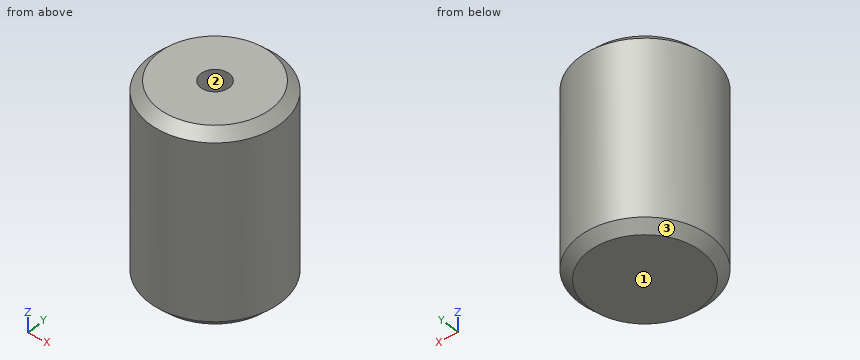
from build123d import *

# Parameters (mm, degrees)
F0_R     = 13.5
F1_DEPTH = 40
F2_R     = 2.9
F3_DEPTH = 35
F4_SIZE  = 2


with BuildPart() as f1:
    # F0 (on Top) → F1 (new body)
    with BuildSketch(Plane.XY):
        Circle(F0_R)
    extrude(amount=F1_DEPTH)

    # F2 (on face) → F3 (cut)
    with BuildSketch(Plane.XY.offset(40)):
        Circle(F2_R)
    extrude(amount=-F3_DEPTH, mode=Mode.SUBTRACT)

    # F4
    f4_edges = [f1.edges().sort_by_distance(p)[0] for p in [
        (-13.5, 0, 0),
        (-13.5, 0, 40),
    ]]
    chamfer(f4_edges, length=F4_SIZE)


solid = f1.part
Geometry check sheet. Reference: the model listing, model coordinates, mm. Face numbers are marked on the shaded views. Give positions to 0.01 mm unless a question says otherwise; leave off trailing zeros. Loops run counter-clockwise (first coordinate to the right, second up) from the corner with the lowest first, then second, coordinate; pieces in that order, holes last. Notation, with made-up numbers: M 10.5,16 L 29.5,16 A8 cw 29.5,24 Z; hole C 74,72.5 d4. An arc over 180 degrees is marked long. Answer as a JSON object with one key per item and string values. Group by question number.
Item 1: Sectioned sample at A-A on y = 0. Record the boundary of the cut face in (x, z).
Item 2: Sectioned sample at B-B on z = 9. Record the boundary of the cut face in (x, y), plus the area to 3 significant figures.
Item 3: Mould release check, pull along Y, two halves, no side actions. Record for the marked faces 1, 2 and 3: pulls with the +Y half, pulls with the -Y half, needs draft (parallel to the pull), parting line crosses it, or undercut.
Item 4: Material ranges on L1, parallel to Y at x = 0, z = 25; L2, parallel to Z at x = 1.75, y = 1.25; L3, parallel to Y at x = -0.75, z = 38, recorded low to high.
Item 5: Gauge pin test, flat ends, axial feed: pin 1 (6.5 mm diameter, centred on x = 0, y = -0.5, fed in from +Z); pin 2 (6 mm diameter, centred on x = 5, z = 30, fed in from +Y); pin 3 (5 mm diameter, centred on x = 0, y = 0, fed in from +Z); pin 4 (3 mm diameter, centred on x = -10.5, z = 31, fed in from -Y). Record the tip position at first contact, or that the pin passes through.
Findings below:
{
 "1": {"outline": "M -13.5,2 L -11.5,0 L 11.5,0 L 13.5,2 L 13.5,38 L 11.5,40 L 2.9,40 L 2.9,5 L -2.9,5 L -2.9,40 L -11.5,40 L -13.5,38 Z"},
 "2": {"outline": "C 0,0 d27; hole C 0,0 d5.8", "area": "546 mm2"},
 "3": {"face 1": "needs draft", "face 2": "undercut", "face 3": "parting line crosses it"},
 "4": {"L1": "-13.5 to -2.9, 2.9 to 13.5", "L2": "0 to 5", "L3": "-13.48 to -2.8, 2.8 to 13.48"},
 "5": {"pin 1": "z = 40", "pin 2": "y = 13.35", "pin 3": "z = 5", "pin 4": "y = -10.06"}
}
